Autodesk Inventor part; units mm, degrees
ref_plane "YZ Plane" through (0, 0, 0) normal (1, 0, 0) x (0, 1, 0)
ref_plane "XZ Plane" through (0, 0, 0) normal (0, 1, 0) x (-1, 0, 0)
ref_plane "XY Plane" through (0, 0, 0) normal (0, 0, 1) x (1, 0, 0)
sketch "Sketch1" plane through (0, 0, 0) normal (0, 1, 0) x (-1, 0, 0)
  line L0 (0, -3.1177) -> (-2.7, -1.5588)
  line L1 (-2.7, -1.5588) -> (-2.7, 1.5588)
  line L2 (-2.7, 1.5588) -> (0, 3.1177)
  line L3 (0, 3.1177) -> (2.7, 1.5588)
  line L4 (2.7, 1.5588) -> (2.7, -1.5588)
  line L5 (2.7, -1.5588) -> (0, -3.1177)
  circle A0 centre (0, 0) radius 1.5
  dimension "d0" = 5.4
  dimension "d1" = 3
extrude "Extrusion1" add sketch "Sketch1" along normal blind 2.4
sketch "Sketch2" plane through (0, 2.4, 0) normal (0, 1, 0) x (1, 0, 0)
  circle A0 centre (0, 0) radius 2.7
  line L0 (2.7, -1.5588) -> (2.7, 1.5588)
  line L1 (-2.7, 1.5588) -> (-2.7, -1.5588)
  circle A1 centre (0, 0) radius 1.5
  dimension "d4" = 5.4
  dimension "d5" = 5.4
extrude "Extrusion2" add sketch "Sketch2" along normal blind 1.4
fillet "Fillet1" radius 0.4 1 edges at (-2.7, 3.8, 0)
equation "\"d5\" = d4"
properties part number "m3_nut_locking" material "Stainless Steel"
Here's how the part is built. I have some questions about the finished solid (model axes, mm). A direction names the side the tool comes from. Coordinates: 2 decimals unless noted, no trailing zeros. Write each loop counter-clockwise with the first axis right and the second up, starting at its lowest first coordinate (ties: lowest second). Pieces come first, ordered by that corner, then holes.
Item 1: I want a section at A-A on y = 1.9. Write out the boundary of the cut face in (x, z).
Item 2: On a 3-axis mill with a long thin cutter (end or side, diameter ignored), from which of +Z, -Z, +X, -X, +Y, -Y can I reach the whole of each face in a straight line? I mean faces 1 (the flat face through (-2.5, 2.4, -1.4)), 2 (the flat face through (-2.5, 2.4, 1.4)), 3 (the flat face through (2.5, 2.4, -1.4)), 4 (the flat face through (2.5, 2.4, 1.4)), 5 (the cylindrical face through (-0.585, 2.893, -2.636)). Say none if no direction works.
Item 3: If I drill on line 1 (X direction, y = 1.9, z = 0); line 2 (Z direction, x = 0.6, y = 0.3), over which ranges is the centre line in solid material (lowest first)?
Item 4: I want a section at B-B on y = 3.3. Write out the boundary of the cut face in (x, z), and give its area (3 significant figures).
Item 5: Will these pins go through, and if not, where does the flat tip stop? pin 1 (0.7 mm diameter, centred on x = 2.5, z = 1, fed in from +Y); pin 2 (1 mm diameter, centred on x = -1.5, y = 2.5, fed in from -Z); pin 3 (2 mm diameter, centred on y = 3.5, z = 2.5, fed in from +X).
Findings below:
1. outline: (-2.7, -1.56) - (0, -3.12) - (2.7, -1.56) - (2.7, 1.56) - (0, 3.12) - (-2.7, 1.56) - close; hole circle Ø3 at (0, 0)
2. face 1: -Z, -X, +Y
2. face 2: +Z, -X, +Y
2. face 3: -Z, +X, +Y
2. face 4: +Z, +X, +Y
2. face 5: +Y
3. line 1: x = -2.7 to -1.5, 1.5 to 2.7
3. line 2: z = -2.77 to -1.37, 1.37 to 2.77
4. outline: circle Ø5.4 at (0, 0); hole circle Ø3 at (0, 0)
4. area: 15.8 mm2
5. pin 1: stops at y = 3.8
5. pin 2: stops at z = -2.53
5. pin 3: stops at x = 2.24
